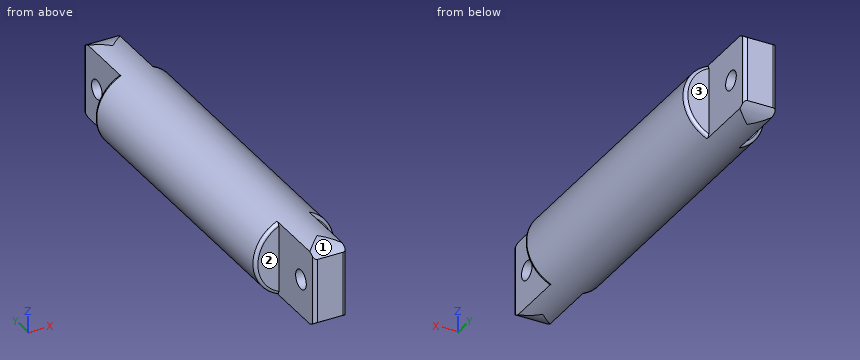
from build123d import *

# Parameters (mm, degrees)
SKETCH1_R              = 124.99999999999999
BOSS_EXTRUDE1_DEPTH    = 650
CUT_EXTRUDE1_START     = -200
CUT_EXTRUDE1_DEPTH     = 200
CUT_EXTRUDE4_START     = -100
CUT_EXTRUDE4_OUTLINE_R = 30
CUT_EXTRUDE4_DEPTH     = 100
FILLET2_R              = 10
FILLET2_OF_MIRROR4_R   = 10
FILLET3_R              = 10
FILLET4_R              = 10


# Read off the part's stored shape, not the designer's step: Cut-Extrude4
with BuildPart() as part:
    # Sketch1 → Boss-Extrude1 (new body)
    with BuildSketch(Plane(origin=(0, 0, 0), x_dir=(1, 0, 0), z_dir=(0, 1, 0))):
        with Locations(Location((0, 0, 0), (0, 0, 270))):
            Circle(SKETCH1_R)
    boss_extrude1 = extrude(amount=BOSS_EXTRUDE1_DEPTH)

    # Sketch2 → Cut-Extrude1 (cut)
    with BuildSketch(Plane(origin=(0, 650, 0), x_dir=(1, 0, 0), z_dir=(0, 1, 0)).offset(CUT_EXTRUDE1_START)):
        with BuildLine():
            Line((-50, -114.56439237389277), (-50, 114.56439237389277))
            ThreePointArc((-50.00000000000426, 114.56439237389412), (-124.99999999999999, 1.531e-14), (-50.00000000000437, -114.56439237389408))
        make_face()
        with BuildLine():
            ThreePointArc((124.99999999999999, 0), (104.5825033167593, 68.46531968814595), (49.999999999999545, 114.56439237389618))
            Line((50, 114.56439237389633), (50, -114.56439237389633))
            ThreePointArc((49.999999999999545, -114.56439237389618), (104.58250331675926, -68.46531968814601), (124.99999999999999, -3.062e-14))
        make_face()
    cut_extrude1 = extrude(amount=CUT_EXTRUDE1_DEPTH, mode=Mode.SUBTRACT)

    # Cut-Extrude4 outline → Cut-Extrude4 (cut)
    with BuildSketch(Plane(origin=(50, 0, 0), x_dir=(0, 0, -1), z_dir=(1, 0, 0)).offset(CUT_EXTRUDE4_START)):
        with BuildLine():
            ThreePointArc((100, 650), (118.585412256, 614.528470752), (125, 575))
            Line((125, 575), (125, 650))
            Line((125, 650), (100, 650))
        make_face()
        with BuildLine():
            Line((-125, 650), (-125, 575))
            ThreePointArc((-125, 575), (-118.585412256, 614.528470752), (-100, 650))
            Line((-100, 650), (-125, 650))
        make_face()
        with Locations((0, 575)):
            Circle(CUT_EXTRUDE4_OUTLINE_R)
    cut_extrude4 = extrude(amount=CUT_EXTRUDE4_DEPTH, mode=Mode.SUBTRACT)

    # Fillet2
    fillet2_edges = [part.edges().sort_by_distance(p)[0] for p in [
        (50, 650, 0),
        (-50, 650, 0),
    ]]
    fillet(fillet2_edges, radius=FILLET2_R)

    # Mirror4: Boss-Extrude1, Cut-Extrude1, Cut-Extrude4 across plane
    add(boss_extrude1.mirror(Plane(origin=(0, 0, 0), x_dir=(0, 0, 1), z_dir=(0, -1, 0))))
    add(cut_extrude1.mirror(Plane(origin=(0, 0, 0), x_dir=(0, 0, 1), z_dir=(0, -1, 0))), mode=Mode.SUBTRACT)
    add(cut_extrude4.mirror(Plane(origin=(0, 0, 0), x_dir=(0, 0, 1), z_dir=(0, -1, 0))), mode=Mode.SUBTRACT)

    # Fillet2 of Mirror4
    fillet2_of_mirror4_edges = [part.edges().sort_by_distance(p)[0] for p in [
        (50, -650, 0),
        (-50, -650, 0),
    ]]
    fillet(fillet2_of_mirror4_edges, radius=FILLET2_OF_MIRROR4_R)

    # Fillet3
    fillet3_edges = [part.edges().sort_by_distance(p)[0] for p in [
        (125, 450, 2.132e-14),
        (-124.99999999999999, 450, -6.04e-14),
    ]]
    fillet(fillet3_edges, radius=FILLET3_R)

    # Fillet4
    fillet4_edges = [part.edges().sort_by_distance(p)[0] for p in [
        (-124.99999999999999, -450, -6.04e-14),
        (125, -450, 2.132e-14),
    ]]
    fillet(fillet4_edges, radius=FILLET4_R)


solid = part.part
Part model, mm, in its own coordinate system. Face numbers are marked on the shaded views. A direction names the side the tool comes from. Round coordinates to 2 decimals unless told otherwise and drop trailing zeros. Loops run counter-clockwise (first coordinate to the right, second up) from the corner with the lowest first, then second, coordinate; pieces in that order, holes last. Notation, with made-up numbers: (-14.5, 81) - (42.5, 81) arc R27 ccw to (42.5, 115) - close; hole circle Ø10 at (28.25, 63.5). An arc over 180 degrees is marked (long way). Answer as a JSON object with one key per item and string values.
Item 1: Wall check: L1, parallel to Y at x = 15.5, z = 0; L2, parallel to Y at x = -45, z = -16; L3, parallel to X at y = 17, z = 0.5. Give the ranges that are in metal, low to high.
Output:
{"L1": "-650 to -605, -545 to 545, 605 to 650", "L2": "-648.66 to -600.38, -549.62 to 549.62, 600.38 to 648.66", "L3": "-125 to 125"}
Item 2: Pin check, flat tips, straight feed: pin 1 (6 mm diameter, centred on y = -470, z = 92, fed in from -X); pin 2 (10 mm diameter, centred on x = -13.5, y = 178.5, fed in from -Z); pin 3 (1.5 mm diameter, centred on y = -84.5, z = -69, fed in from -X). Stop position of each tip, or through.
Output:
{"pin 1": "x = -50", "pin 2": "z = -124.71", "pin 3": "x = -104.72"}
Item 3: Tool access for the marked faces 1, 2 and 3: list every direction of +Z, -Z, +X, -X, +Y, -Y with a clear straight run to the whole face (end or side of a thin tool).
Output:
{"face 1": "+Z, +X, -X, -Y", "face 2": "+Z, -Z, -X, -Y", "face 3": "+Z, -Z, +X, +Y"}
Item 4: Band-saw the part on B-B on y = -168.5. List the corners of the cut face in (x, z), plus the area to 3 significant figures.
Output:
{"outline": "circle Ø250 at (0, 0)", "area": "49,100 mm2"}
Item 5: Band-saw the part on A-A on z = 0. List the corners of the cut face in (x, y).
Output:
{"outline": "(-125, -440) arc R10 ccw to (-115, -450) - (-50, -450) - (-50, -545) - (50, -545) - (50, -450) - (115, -450) arc R10 ccw to (125, -440) - (125, 440) arc R10 ccw to (115, 450) - (50, 450) - (50, 545) - (-50, 545) - (-50, 450) - (-115, 450) arc R10 ccw to (-125, 440) - close; (-50, -640) arc R10 ccw to (-40, -650) - (40, -650) arc R10 ccw to (50, -640) - (50, -605) - (-50, -605) - close; (-50, 605) - (50, 605) - (50, 640) arc R10 ccw to (40, 650) - (-40, 650) arc R10 ccw to (-50, 640) - close"}
Item 6: Band-saw the part on C-C on y = -516. List the corners of the cut face in (x, z), plus the area to 3 significant figures.
Output:
{"outline": "(-50, -114.56) arc R125 ccw to (50, -114.56) - (50, 114.56) arc R125 ccw to (-50, 114.56) - close", "area": "24,300 mm2"}
